Source: CAD feature listing. Evaluate the final solid. Frame: model axes, mm. A direction names the side the tool comes from. Give positions to 0.01 mm unless a question says otherwise; leave off trailing zeros. Loops run counter-clockwise (first coordinate to the right, second up) from the corner with the lowest first, then second, coordinate; pieces in that order, holes last.
```python
from build123d import *

# Parameters (mm, degrees)
SKETCH1_W           = 355.6
SKETCH1_H           = 355.6
BOSS_EXTRUDE1_DEPTH = 100
FILLET1_R           = 70
SKETCH2_R           = 7.03
CUT_EXTRUDE1_DEPTH  = 25.04
FILLET3_R           = 5
FILLET4_R           = 10
SKETCH3_R           = 15
BOSS_EXTRUDE2_DEPTH = 17.7


with BuildPart() as part:
    # Sketch1 → Boss-Extrude1 (new body)
    with BuildSketch(Plane.XY):
        Rectangle(SKETCH1_W, SKETCH1_H)
    extrude(amount=BOSS_EXTRUDE1_DEPTH)

    # Fillet1
    fillet1_edges = [part.edges().sort_by_distance(p)[0] for p in [
        (-177.8, -177.8, 50),
        (-177.8, 177.8, 50),
        (177.8, 177.8, 50),
        (177.8, -177.8, 50),
    ]]
    fillet(fillet1_edges, radius=FILLET1_R)

    # Sketch2 → Cut-Extrude1 (cut)
    with BuildSketch(Plane.XY.offset(100)):
        with Locations((-104.42, -125.46)):
            Circle(SKETCH2_R)
    extrude(amount=-CUT_EXTRUDE1_DEPTH, mode=Mode.SUBTRACT)

    # Fillet3
    fillet3_edges = [part.edges().sort_by_distance(p)[0] for p in [
        (0, 177.8, 0),
        (177.8, 0, 0),
        (0, -177.8, 0),
        (-177.8, 0, 0),
        (-157.297474683, 157.297474683, 0),
        (-157.297474683, -157.297474683, 0),
        (157.297474683, -157.297474683, 0),
        (157.297474683, 157.297474683, 0),
    ]]
    fillet(fillet3_edges, radius=FILLET3_R)

    # Fillet4
    fillet4_edges = [part.edges().sort_by_distance(p)[0] for p in [
        (0, 177.8, 100),
        (177.8, 0, 100),
        (-177.8, 0, 100),
        (0, -177.8, 100),
        (-157.297474683, 157.297474683, 100),
        (-157.297474683, -157.297474683, 100),
        (157.297474683, -157.297474683, 100),
        (157.297474683, 157.297474683, 100),
    ]]
    fillet(fillet4_edges, radius=FILLET4_R)

    # Sketch3 → Boss-Extrude2 (add)
    with BuildSketch(Plane.XY.offset(100)):
        Circle(SKETCH3_R)
    extrude(amount=BOSS_EXTRUDE2_DEPTH)


solid = part.part
```
(1) Mould query, pull axis Y, two halves, no side actions, for faces 1 (the flat face through (177.8, -2, 47)), 2 (the cylindrical face through (-1.51, -174.79, 97.15)), 3 (the cylindrical face through (-109.6, -120.71, 87.66)). Classes: pulls with the +Y half, pulls with the -Y half, needs draft (parallel to the pull), parting line crosses it, or undercut.
A:
face 1: needs draft
face 2: pulls with the -Y half
face 3: undercut
(2) Reachability of faces 4 (the cylindrical face through (-14.985, 0.66, 108.726)), 5 (the cylindrical face through (157.84, 156.75, 48.1)) from +Z, -Z, +X, -X, +Y, -Y: full face, straight path, thin tool, end or side. Return the list, or none.
A:
face 4: +Z
face 5: +Z, -Z, +X, +Y
(3) Ray query, line 1 along Y through (x, z) = (-104.42, 80); line 2 along Z through (x, y) = (-105, 42); line 3 along X through (y, z) = (-125, 87). Return the intervals inside material, ascending.
A:
line 1: y = -177.8 to -132.49, -118.43 to 177.8
line 2: z = 0 to 100
line 3: x = -175.65 to -111.43, -97.41 to 175.65
(4) First-contact query: pin 1 (18.5 mm diameter, centred on x = -104.42, y = -125.46, fed in from +Z); pin 2 (4 mm diameter, centred on x = -117, z = 53.5, fed in from +Y); pin 3 (7 mm diameter, centred on x = -104.5, y = -122.5, fed in from +Z); pin 4 (1.5 mm diameter, centred on y = 130, z = 102.5, fed in from -X). Flat tips, straight axial feed; report the tip coordinate or a pass-through.
A:
pin 1: stops at z = 100
pin 2: stops at y = 177.43
pin 3: stops at z = 74.96
pin 4: passes through
(5) Section A-A, the plane z = 59. Return the cut outline in (x, y).
A:
outline: (-177.8, -107.8) arc R70 ccw to (-107.8, -177.8) - (107.8, -177.8) arc R70 ccw to (177.8, -107.8) - (177.8, 107.8) arc R70 ccw to (107.8, 177.8) - (-107.8, 177.8) arc R70 ccw to (-177.8, 107.8) - close
(6) Section B-B, the plane y = 0. Return the cut outline in (x, z), then the cut area to 3 significant figures.
A:
outline: (-177.8, 5) arc R5 ccw to (-172.8, 0) - (172.8, 0) arc R5 ccw to (177.8, 5) - (177.8, 90) arc R10 ccw to (167.8, 100) - (15, 100) - (15, 117.7) - (-15, 117.7) - (-15, 100) - (-167.8, 100) arc R10 ccw to (-177.8, 90) - close
area: 36,000 mm2
(7) Section D-D, the plane y = 75. Return the cut outline in (x, z), then the cut area to 3 significant figures.
A:
outline: (-177.8, 5) arc R5 ccw to (-172.8, 0) - (172.8, 0) arc R5 ccw to (177.8, 5) - (177.8, 90) arc R10 ccw to (167.8, 100) - (-167.8, 100) arc R10 ccw to (-177.8, 90) - close
area: 35,500 mm2
